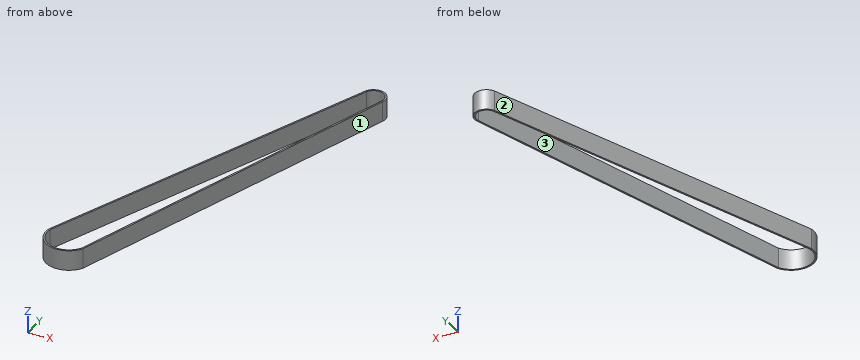
Autodesk Inventor part; units mm, degrees
ref_plane "YZ Plane" through (0, 0, 0) normal (1, 0, 0) x (0, 1, 0)
ref_plane "XZ Plane" through (0, 0, 0) normal (0, 1, 0) x (-1, 0, 0)
ref_plane "XY Plane" through (0, 0, 0) normal (0, 0, 1) x (1, 0, 0)
ref_plane "Work Plane1" through (0, 0, 0) normal (0, 0, 1) x (1, 0, 0)
sketch "Sketch1" plane through (0, 0, 0) normal (0, 0, 1) x (1, 0, 0)
  arc A0 (7.5768, -31.9111) -> (11.0096, -30.8953) centre (0, 0) ccw construction
  arc A1 (2.7361, -32.684) -> (6.282, -32.1911) centre (0, 0) ccw construction
  arc A2 (-2.1658, -32.7267) -> (1.414, -32.7678) centre (0, 0) ccw construction
  arc A3 (12.2483, -30.4254) -> (15.4914, -28.9093) centre (0, 0) ccw construction
  arc A4 (16.6462, -28.2601) -> (19.627, -26.2775) centre (0, 0) ccw construction
  circle A5 centre (0, 0) radius 37.1131 construction
  circle A6 centre (0, 0) radius 32.4639 construction
  arc A7 (-32.3268, 5.5412) -> (28.3967, -16.412) centre (0, 0) ccw
  circle A8 centre (185.9759, 522.491) radius 15.875 construction
  circle A9 centre (185.9759, 522.491) radius 6.35 construction
  arc A10 (198.6184, 512.8898) -> (171.693, 529.4203) centre (185.9759, 522.491) ccw construction
  arc A11 (200.9863, 517.3234) -> (171.693, 529.4203) centre (185.9759, 522.491) ccw
  line L0 (200.9863, 517.3234) -> (28.3967, -16.412)
  line L1 (-32.3268, 5.5412) -> (171.693, 529.4203)
  arc A12 (203.396, 516.52) -> (169.3619, 530.4337) centre (185.9759, 522.491) ccw
  line L2 (203.396, 516.52) -> (30.7322, -17.445)
  arc A13 (-34.7852, 6.228) -> (30.7322, -17.445) centre (0, 0) ccw
  line L3 (-34.7852, 6.228) -> (169.3619, 530.4337)
  dimension "d0" = 2.54
extrude "Extrusion1" add sketch "Sketch1" along normal up to surface (30.8991 mm away)
properties part number "Belt" material "Acetal Resin, Black"
Design review of the part built by this model. Coordinates are the model's own, in mm. Face numbers are marked on the shaded views. Coordinates: 2 decimals unless noted, no trailing zeros. Order: outer loops, then holes, each group sorted by start corner. A loop starts at its lowest first (then second) coordinate and runs counter-clockwise, first axis right, second up. Notation, with made-up numbers: M 16.25,34.25 L 48.25,34.25 A35 ccw 48.25,70.25 Z; hole C 0.5,-19.5 d11. An arc over 180 degrees is marked long. Answer as a JSON object with one key per item and string values. Group by question number.
1) Add section B-B, the plane x = 138. Write out the cut boundary in (y, z), then the cut area to 3 significant figures.
2) For pin 1 (6 mm diameter, centred on y = 451, z = 17, fed in from +X); pin 2 (5 mm diameter, centred on y = 48, z = 16, fed in from +X); pin 3 (4 mm diameter, centred on y = 424.5, z = 14, fed in from +X), all flat-tipped, find the tip position at first contact; note any pin that passes through.
3) Mouldability with a two-part tool opening along X and no side actions: class the marked faces 1, 2 and 3 as pulls with the +X half, pulls with the -X half, needs draft (parallel to the pull), parting line crosses it, or undercut.
4) Add section A-A, the plane z = 10.5. Write out the cut boundary in (x, y) (3 decimals).
5) Wall thickness on L1, parallel to X at y = 471, z = 12.5; L2, parallel to X at y = 164, z = 5: over which ranges is each line inside the solid? List them lowest first.
6) Add section C-C, the plane y = 26.5. Write out the cut boundary in (x, z), then the cut area to 3 significant figures.
Computed values:
{
 "1": {"outline": "M 314.28,0 L 322.54,0 L 322.54,30.9 L 314.28,30.9 Z; M 442.9,0 L 449.9,0 L 449.9,30.9 L 442.9,30.9 Z", "area": "471 mm^2"},
 "2": {"pin 1": "stops at x = 183.18", "pin 2": "stops at x = 52.7", "pin 3": "stops at x = 174.29"},
 "3": {"face 1": "pulls with the +X half", "face 2": "pulls with the -X half", "face 3": "undercut"},
 "4": {"outline": "M -34.785,6.228 A35.338 ccw 30.732,-17.445 L 203.396,516.52 A18.415 ccw 169.362,530.434 Z; hole M -32.327,5.541 A32.798 ccw 28.397,-16.412 L 200.986,517.323 A15.875 ccw 171.693,529.42 Z"},
 "5": {"L1": "x = 146.22 to 148.94, 186.01 to 188.68", "L2": "x = 26.66 to 29.38, 86.74 to 89.4"},
 "6": {"outline": "M -26.89,0 L -24.16,0 L -24.16,30.9 L -26.89,30.9 Z; M 42.27,0 L 44.94,0 L 44.94,30.9 L 42.27,30.9 Z", "area": "167 mm^2"}
}
